```python
from build123d import *

# Parameters (mm, degrees)
SKETCH1_W               = 62
SKETCH1_H               = 70
SKETCH1_R               = 8.75
BOTTOM_DEPTH            = 4
SKETCH2_R               = 3.25
SKETCH2_R_2             = 3.75
SCREW_INLETS_DEPTH      = 2.3
SKETCH3_R               = 2.1
MOUNTING_ARMS_DEPTH     = 4
WALLS_DEPTH             = 22
ADAPTER_BOLT_HOLE_REACH = 102.081
SKETCH5_R               = 4
M2_LOCK_HOLES_REACH     = 96.241
SKETCH7_R               = 1.25


with BuildPart() as part:
    # Sketch1 → Bottom (new body)
    with BuildSketch(Plane.XY):
        with Locations((21, 17)):
            Rectangle(SKETCH1_W, SKETCH1_H)
        with Locations((21, 21)):
            Circle(SKETCH1_R, mode=Mode.SUBTRACT)
    extrude(amount=BOTTOM_DEPTH)

    # Sketch2 → Screw_inlets (cut)
    with BuildSketch(Plane(origin=(0, 0, 0), x_dir=(-1, 0, 0), z_dir=(0, 0, -1))):
        with Locations((-37.5, 4.5)):
            Circle(SKETCH2_R)
        with Locations((-37.5, 37.5)):
            Circle(SKETCH2_R)
        with Locations((-27, 4)):
            Circle(SKETCH2_R_2)
        with Locations((-15, 4)):
            Circle(SKETCH2_R_2)
        with Locations((-4.5, 4.5)):
            Circle(SKETCH2_R)
        with Locations((-4.5, 37.5)):
            Circle(SKETCH2_R)
    extrude(amount=-SCREW_INLETS_DEPTH, mode=Mode.SUBTRACT)

    # Sketch3 → Mounting_arms (add)
    # profile 1 of 4: a face of its own
    with BuildSketch(Plane(origin=(0, 0, 0), x_dir=(-1, 0, 0), z_dir=(0, 0, -1))):
        with BuildLine():
            Line((10, 40.688384135), (18.929587578, 50.770176561))
            ThreePointArc((18.929587578, 50.770176561), (18.287940566, 61.357352252), (7.700764875, 60.715705241))
            Line((7.700764875, 60.715705241), (-0.018859766, 52))
            Line((-0.018859766, 52), (10, 52))
            Line((10, 52), (10, 40.688384135))
        make_face()
        with Locations((13.315176226, 55.742940901)):
            Circle(SKETCH3_R, mode=Mode.SUBTRACT)
    # profile 2 of 4: a face of its own
    with BuildSketch(Plane(origin=(0, 0, 0), x_dir=(-1, 0, 0), z_dir=(0, 0, -1))):
        with BuildLine():
            Line((-52, 40.688384135), (-60.929587578, 50.770176561))
            ThreePointArc((-60.929587578, 50.770176561), (-60.287940566, 61.357352252), (-49.700764875, 60.715705241))
            Line((-49.700764875, 60.715705241), (-41.981140234, 52))
            Line((-41.981140234, 52), (-52, 52))
            Line((-52, 52), (-52, 40.688384135))
        make_face()
        with Locations((-55.315176226, 55.742940901)):
            Circle(SKETCH3_R, mode=Mode.SUBTRACT)
    # profile 3 of 4: a face of its own
    with BuildSketch(Plane(origin=(0, 0, 0), x_dir=(-1, 0, 0), z_dir=(0, 0, -1))):
        with BuildLine():
            Line((10, -6.688384135), (18.929587578, -16.770176561))
            ThreePointArc((18.929587578, -16.770176561), (18.287940566, -27.357352252), (7.700764875, -26.715705241))
            Line((7.700764875, -26.715705241), (-0.018859766, -18))
            Line((-0.018859766, -18), (10, -18))
            Line((10, -18), (10, -6.688384135))
        make_face()
        with Locations((13.315176226, -21.742940901)):
            Circle(SKETCH3_R, mode=Mode.SUBTRACT)
    # profile 4 of 4: a face of its own
    with BuildSketch(Plane(origin=(0, 0, 0), x_dir=(-1, 0, 0), z_dir=(0, 0, -1))):
        with BuildLine():
            Line((-52, -18), (-52, -6.688384135))
            Line((-52, -6.688384135), (-60.929587578, -16.770176561))
            ThreePointArc((-60.929587578, -16.770176561), (-60.287940566, -27.357352252), (-49.700764875, -26.715705241))
            Line((-49.700764875, -26.715705241), (-41.981140234, -18))
            Line((-41.981140234, -18), (-52, -18))
        make_face()
        with Locations((-55.315176226, -21.742940901)):
            Circle(SKETCH3_R, mode=Mode.SUBTRACT)
    extrude(amount=-MOUNTING_ARMS_DEPTH)

    # Sketch4 → Walls (add)
    with BuildSketch(Plane(origin=(0, 0, 0), x_dir=(-1, 0, 0), z_dir=(0, 0, -1))):
        Polygon((-6.5, -11.5), (-35.5, -11.5), (-35.5, -3.5), (-45.5, -3.5), (-45.5, 45.5), (3.5, 45.5), (3.5, -3.5), (-6.5, -3.5), align=None)
        Polygon((-9.5, -8.5), (-32.5, -8.5), (-32.5, -0.5), (-42.5, -0.5), (-42.5, 42.5), (0.5, 42.5), (0.5, -0.5), (-9.5, -0.5), align=None, mode=Mode.SUBTRACT)
    extrude(amount=WALLS_DEPTH)

    # Sketch5 → Adapter_bolt_hole (cut, up to next)
    with BuildSketch(Plane.XZ.offset(11.5), mode=Mode.PRIVATE) as adapter_bolt_hole_sk1:
        with Locations(Location((21, -8.5, 0), (0, 0, 270))):
            Circle(SKETCH5_R)
    adapter_bolt_hole_tool1 = extrude(adapter_bolt_hole_sk1.sketch, amount=-ADAPTER_BOLT_HOLE_REACH, mode=Mode.PRIVATE) & part.part
    add(adapter_bolt_hole_tool1.solids().sort_by_distance((21, -11.5, -8.5))[0], mode=Mode.SUBTRACT)

    # M2_lock_holes: up to this face of the body (flat: up to its plane)
    m2_lock_holes_end = Plane(part.part.faces().sort_by_distance((-3.5, 21, -11))[0])
    # Sketch7 → M2_lock_holes (cut, up to the picked face)
    with BuildSketch(Plane(origin=(45.5, 0, 0), x_dir=(0, 0, -1), z_dir=(1, 0, 0)), mode=Mode.PRIVATE) as m2_lock_holes_sk1:
        with Locations(Location((19.25, 28, 0), (0, 0, 90))):
            Circle(SKETCH7_R)
    m2_lock_holes_tool1 = split(extrude(m2_lock_holes_sk1.sketch, amount=-M2_LOCK_HOLES_REACH, mode=Mode.PRIVATE), bisect_by=m2_lock_holes_end, keep=Keep.BOTH, mode=Mode.PRIVATE)
    # Sketch7 → M2_lock_holes (cut, up to the picked face)
    with BuildSketch(Plane(origin=(45.5, 0, 0), x_dir=(0, 0, -1), z_dir=(1, 0, 0)), mode=Mode.PRIVATE) as m2_lock_holes_sk2:
        with Locations(Location((19.25, 14, 0), (0, 0, 90))):
            Circle(SKETCH7_R)
    m2_lock_holes_tool2 = split(extrude(m2_lock_holes_sk2.sketch, amount=-M2_LOCK_HOLES_REACH, mode=Mode.PRIVATE), bisect_by=m2_lock_holes_end, keep=Keep.BOTH, mode=Mode.PRIVATE)
    add(m2_lock_holes_tool1.solids().sort_by(Axis((45.5, 28, -19.25), (-1, 0, 0)))[0], mode=Mode.SUBTRACT)
    add(m2_lock_holes_tool2.solids().sort_by(Axis((45.5, 14, -19.25), (-1, 0, 0)))[0], mode=Mode.SUBTRACT)


solid = part.part
```
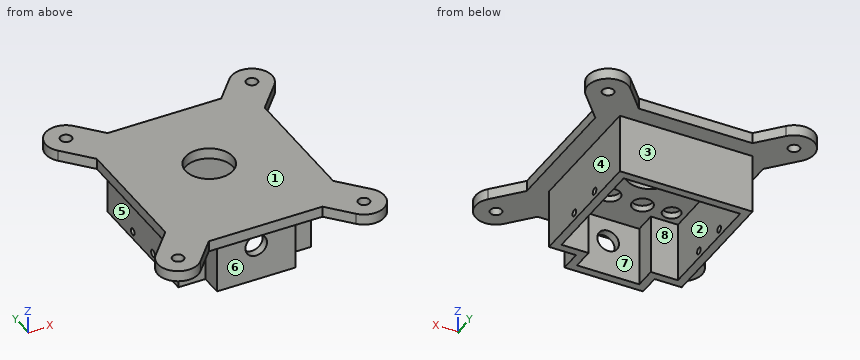
Check sheet for the modelled part. Datum: model origin and axes. Units: mm. Face numbers are marked on the shaded views. A direction names the side the tool comes from. Give positions to 0.01 mm unless a question says otherwise; leave off trailing zeros. Loops run counter-clockwise (first coordinate to the right, second up) from the corner with the lowest first, then second, coordinate; pieces in that order, holes last. Notation, with made-up numbers: (-38.75, 34) - (-16.75, 34) arc R13 cw to (-16.75, 57) - close; hole circle Ø1 at (40.25, 82). An arc over 180 degrees is marked (long way). One line per question, with ' | ' between items. Start each with the question number.
1. Cross-section at B-B, the plane x = 37.5. Enter the section's corners in (y, z), plus the area to 3 significant figures.
2. Material ranges on line 1 along Y through (x, z) = (37.5, 1.4); line 2 along X through (y, z) = (28.5, -17.5); line 3 along Y through (x, z) = (25, -18), recorded low to high. Write a range as [from, to].
3. Set-up check for the marked faces 1, 2, 3 and 4: record each of +Z, -Z, +X, -X, +Y, -Y from which the full face is reachable in a straight line by a thin tool's end or side.
4. Draft check along X on the marked faces 5, 6, 7 and 8. Enter one of: released by +X, released by -X, zero draft, split by the parting line, or undercut.
5. Gauge pin test, flat ends, axial feed: pin 1 Ø12 at (x, z) = (40, -16) entering from -Y; pin 2 Ø11 at (x, z) = (24.5, -12) entering from +Y; pin 3 Ø4.5 at (y, z) = (23.5, 1.5) entering from -X; pin 4 Ø10 at (x, y) = (40.5, 37) entering from -Z. Record the tip position at first contact, or that the pin passes through.
6. Cross-section at A-A, the plane y = 21. Enter the section's corners in (x, z), plus the area to 3 significant figures.
7. Cross-section at C-C, the plane y = 37.5. Enter the section's corners in (x, z).
Check result:
1) outline: (-18, 0) - (-3.5, 0) - (-3.5, -22) - (-0.5, -22) - (-0.5, 0) - (1.25, 0) - (1.25, 2.3) - (7.75, 2.3) - (7.75, 0) - (34.25, 0) - (34.25, 2.3) - (40.75, 2.3) - (40.75, 0) - (42.5, 0) - (42.5, -22) - (45.5, -22) - (45.5, 0) - (52, 0) - (52, 4) - (-18, 4) - close | area: 382 mm2
2) line 1: y = [-18, 1.25], [7.75, 34.25], [40.75, 52] | line 2: x = [-3.5, -0.5], [42.5, 45.5] | line 3: y = [-11.5, -8.5], [42.5, 45.5]
3) face 1: +Z, +X, -X, +Y, -Y | face 2: -Z | face 3: -Z, +X, -X, +Y | face 4: -Z, +X, +Y, -Y
4) face 5: released by -X | face 6: zero draft | face 7: undercut | face 8: undercut
5) pin 1: stops at y = -11.5 | pin 2: stops at y = 45.5 | pin 3: stops at x = -10 | pin 4: stops at z = -22
6) outline: (-10, 0) - (-3.5, 0) - (-3.5, -22) - (-0.5, -22) - (-0.5, 0) - (12.25, 0) - (12.25, 4) - (-10, 4) - close; (29.75, 0) - (42.5, 0) - (42.5, -22) - (45.5, -22) - (45.5, 0) - (52, 0) - (52, 4) - (29.75, 4) - close | area: 310 mm2
7) outline: (-10, 0) - (-3.5, 0) - (-3.5, -22) - (-0.5, -22) - (-0.5, 0) - (1.25, 0) - (1.25, 2.3) - (7.75, 2.3) - (7.75, 0) - (34.25, 0) - (34.25, 2.3) - (40.75, 2.3) - (40.75, 0) - (42.5, 0) - (42.5, -22) - (45.5, -22) - (45.5, 0) - (52, 0) - (52, 4) - (-10, 4) - close
